```python
from build123d import *

# Parameters (mm, degrees)
SKETCH_1_R          = 2.2
SKETCH_1_R_2        = 2.7
EXTRUDE_1_DEPTH     = 5
CUT_EXTRUDE_1_REACH = 59.46
EXTRUDE_START       = -5
SKETCH_6_R          = 2.7
EXTRUDE_3_DEPTH     = 5
FILLET_1_R          = 5


with BuildPart() as part:
    # 草图1 → 凸台-拉伸1 (new body)
    with BuildSketch(Plane.XY):
        with BuildLine():
            Line((-21.928513003, 31.619793089), (-45, 12.5))
            Line((-45, 12.5), (-45, -12.5))
            Line((-45, -12.5), (-21.928513003, -31.619793089))
            ThreePointArc((-21.928513003, -31.619793089), (-18.386291168, -32.993165888), (-14.729286549, -31.963697294))
            Line((-14.729286549, -31.963697294), (22.594284602, -6.618263059))
            ThreePointArc((22.594284602, -6.618263059), (26.1, 0), (22.594284602, 6.618263059))
            Line((22.594284602, 6.618263059), (-14.729286549, 31.963697294))
            ThreePointArc((-14.729286549, 31.963697294), (-18.386291168, 32.993165888), (-21.928513003, 31.619793089))
        make_face()
        with Locations((-34.1, 0)):
            Circle(SKETCH_1_R, mode=Mode.SUBTRACT)
        with Locations((-18.1, 27)):
            Circle(SKETCH_1_R_2, mode=Mode.SUBTRACT)
        with Locations((-18.1, -27)):
            Circle(SKETCH_1_R_2, mode=Mode.SUBTRACT)
        with Locations((18.1, 0)):
            Circle(SKETCH_1_R_2, mode=Mode.SUBTRACT)
    extrude(amount=EXTRUDE_1_DEPTH)

    # 草图4 → 旋转1 (revolve)
    with BuildSketch(Plane(origin=(-24.93598604, 16.933358057, 0), x_dir=(0, 0, -1), z_dir=(0.8272828823621655, -0.5617855752425007, 0)), mode=Mode.PRIVATE) as revolve_1_sk:
        Polygon((8.7, 17.168318912), (8.7, 14.868318912), (0, 14.868318912), (0, 18.168318912), align=None)
    revolve_1 = revolve(revolve_1_sk.sketch.rotate(Axis((-18.1, 27, 1000.278995542), (0, 0, -1)), 55.820627671), axis=Axis((-18.1, 27, 1000.278995542), (0, 0, -1)))

    # 镜向1: 旋转1 across plane
    add(revolve_1.mirror(Plane.ZX))

    # 草图5 → 切除-拉伸1 (cut, up to next)
    with BuildSketch(Plane.XY.offset(5), mode=Mode.PRIVATE) as cut_extrude_1_sk1:
        with BuildLine():
            Line((-24.1, -27), (-24.1, 27))
            ThreePointArc((-24.1, 27), (-23.53005884, 29.552344215), (-21.928513003, 31.619793089))
            Line((-21.928513003, 31.619793089), (-45, 12.5))
            Line((-45, 12.5), (-45, -12.5))
            Line((-45, -12.5), (-21.928513003, -31.619793089))
            ThreePointArc((-21.928513003, -31.619793089), (-23.53005884, -29.552344215), (-24.1, -27))
        make_face()
    cut_extrude_1_tool1 = extrude(cut_extrude_1_sk1.sketch, amount=-CUT_EXTRUDE_1_REACH, mode=Mode.PRIVATE) & part.part
    add(cut_extrude_1_tool1.solids().sort_by_distance((-33.100815, 0, 5))[0], mode=Mode.SUBTRACT)

    # 草图6 → 凸台-拉伸3 (add)
    with BuildSketch(Plane.XY.offset(5).offset(EXTRUDE_START)):
        Polygon((12.5, -13.473020485), (-14.729286549, -31.963697294), (23.5, -31.963697294), (23.5, 31.963697294), (-14.729286549, 31.963697294), (12.5, 13.473020485), align=None)
        with Locations((18.1, 0)):
            Circle(SKETCH_6_R, mode=Mode.SUBTRACT)
    extrude(amount=EXTRUDE_3_DEPTH)

    # 草图7 → 旋转2 (revolve)
    with BuildSketch(Plane(origin=(6.469864276, 8.674410623, 0), x_dir=(0.8015915013283047, -0.5978721142503927, 0), z_dir=(0.5978721142503927, 0.8015915013283047, 0)), mode=Mode.PRIVATE) as revolve_2_sk:
        Polygon((11.808806174, 8.7), (11.808806174, 0), (8.508806174, 0), (9.508806174, 8.7), align=None)
    revolve(revolve_2_sk.sketch.rotate(Axis((18.1, 0, 1), (0, 0, -1)), 143.282349417), axis=Axis((18.1, 0, 1), (0, 0, -1)))

    # 圆角1
    fillet_1_edges = [part.edges().sort_by_distance(p)[0] for p in [
        (23.5, 31.963697294, 2.5),
        (23.5, -31.963697294, 2.5),
    ]]
    fillet(fillet_1_edges, radius=FILLET_1_R)


solid = part.part
```
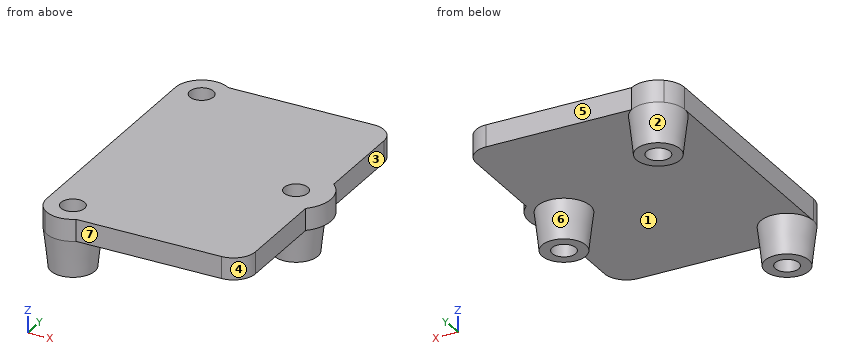
Verification items for the finished model (mm, model axes). Face numbers are marked on the shaded views. A direction names the side the tool comes from. Coordinates: 2 decimals unless noted, no trailing zeros. Loops run counter-clockwise (first coordinate to the right, second up) from the corner with the lowest first, then second, coordinate; pieces in that order, holes last. Notation, with made-up numbers: (71, 40) -> (115, 40) arc R25 cw to (115, 60) -> close; hole circle Ø5 at (-2.75, 66). An arc over 180 degrees is marked (long way). Answer in a Markdown table with one row per item. Add a question column.
1. Section check A-A, the plane x = -18.1. Enter the section's corners in (y, z).
2. Section check B-B, the plane y = 0. Enter the section's corners in (x, z).
3. Access from +Z, -Z, +X, -X, +Y, -Y to the whole of each face (thin tool, end or side, straight path). Record for the marked faces 5, 6 and 7.
4. Section check C-C, the plane z = -2.75. Enter the section's corners in (x, y), then the cut area to 3 significant figures.
5. Material ranges on probe 1 along Y at (x, z) = (-18.1, 3.6); probe 2 along Z at (x, y) = (9.5, 1); probe 3 along Y at (x, z) = (6.5, 0.25), recorded low to high. Write a range as [from, to].
6. Draft check along Y on the marked faces 1, 2, 3 and 4. Enter one of: +Y half, -Y half, draft (parallel to the pull), parting line (faces both ways), or undercut.
7. Depth check by flat-ended pin: P1, Ø3, axis at x = 18.1, y = 0, coming from the -Z side; P2, Ø2, axis at x = 4, z = 2, coming from the +Y side; P3, Ø5.5, axis at y = 12.5, z = 3, coming from the +X side; P4, Ø4, axis at x = -5.5, z = 3.5, coming from the -Y side. Enter the tip coordinate at first touch or a pass-through.
8. Section check D-D, the plane z = -6.25. Enter the section's corners in (x, y), then the cut area to 3 significant figures.
Derived:
| question | item | result |
|---|---|---|
| 1 | outline | (-33, 0) -> (-32, -8.7) -> (-29.7, -8.7) -> (-29.7, 5) -> (-33, 5) -> close; (-24.3, -8.7) -> (-22, -8.7) -> (-21, 0) -> (21, 0) -> (22, -8.7) -> (24.3, -8.7) -> (24.3, 5) -> (-24.3, 5) -> close; (29.7, -8.7) -> (32, -8.7) -> (33, 0) -> (33, 5) -> (29.7, 5) -> close |
| 2 | outline | (-24.1, 0) -> (12.1, 0) -> (13.1, -8.7) -> (15.4, -8.7) -> (15.4, 5) -> (-24.1, 5) -> close; (20.8, -8.7) -> (23.1, -8.7) -> (24.1, 0) -> (26.1, 0) -> (26.1, 5) -> (20.8, 5) -> close |
| 3 | face 5 | +Z, -Z, +X, +Y |
| 3 | face 6 | -Z |
| 3 | face 7 | +Z, -Z, +X, -Y |
| 4 | outline | circle Ø11.37 at (-18.1, -27); circle Ø11.37 at (-18.1, 27); circle Ø11.37 at (18.1, 0); hole circle Ø5.4 at (-18.1, -27); hole circle Ø5.4 at (-18.1, 27); hole circle Ø5.4 at (18.1, 0) |
| 4 | area | 236 mm² |
| 5 | probe 1 | y = [-33, -29.7], [-24.3, 24.3], [29.7, 33] |
| 5 | probe 2 | z = [0, 5] |
| 5 | probe 3 | y = [-31.96, 31.96] |
| 6 | face 1 | undercut |
| 6 | face 2 | undercut |
| 6 | face 3 | draft |
| 6 | face 4 | -Y half |
| 7 | P1 | passes through |
| 7 | P2 | stops at y = 31.96 |
| 7 | P3 | stops at x = 23.5 |
| 7 | P4 | stops at y = -31.96 |
| 8 | outline | circle Ø10.56 at (-18.1, -27); circle Ø10.56 at (-18.1, 27); circle Ø10.56 at (18.1, 0); hole circle Ø5.4 at (-18.1, -27); hole circle Ø5.4 at (-18.1, 27); hole circle Ø5.4 at (18.1, 0) |
| 8 | area | 194 mm² |
